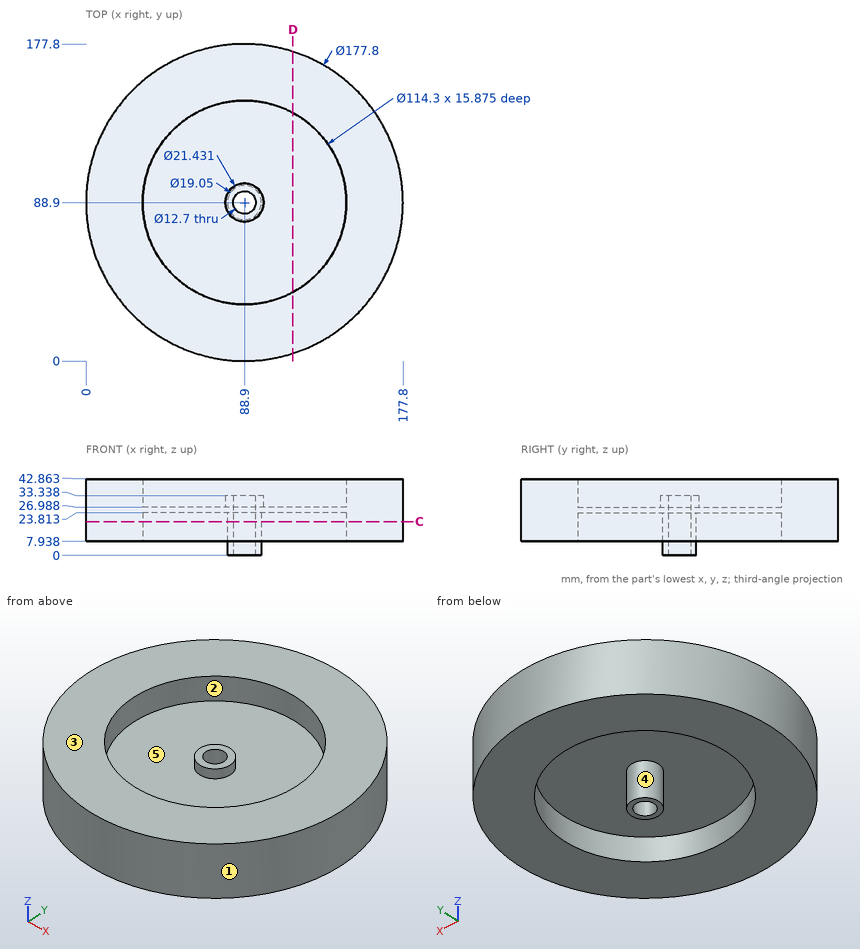
Geometry check sheet. Reference: drawing and pictorial views, mm from the part's lowest x, y, z. A direction names the side the tool comes from. Coordinates: 2 decimals unless noted, no trailing zeros. Loops run counter-clockwise (first coordinate to the right, second up) from the corner with the lowest first, then second, coordinate; pieces in that order, holes last. Notation, with made-up numbers: (-16, 60.5) -> (-7, 60.5) arc R19 cw to (-7, 68.5) -> close; hole circle Ø3 at (48, 83.5). An arc over 180 degrees is marked (long way). Write item = value, one per line. Start each with the question number.
1. Material ranges on line 1 (X direction, y = 88, z = 35) (1 decimal); line 2 (X direction, y = 88, z = 17) (1 decimal); line 3 (Y direction, x = 88.9, z = 33.5), recorded low to high.
2. Tool access check on the marked faces 4 and 5. Record the directions out of +Z, -Z, +X, -X, +Y, -Y that give a thin tool (end or side, any length) a straight path to the whole face; none if there is none.
3. Depth check by flat-ended pin: P1, Ø1, axis at y = 41, z = 11.5, coming from the -X side; P2, Ø8, axis at x = 76, z = 20.5, coming from the +Y side; P3, Ø5, axis at x = 48, y = 50, coming from the -Z side. Enter the tip coordinate at first touch or a pass-through.
4. Section check C-C on z = 19. Give the number of separate pieces and of enclosed holes in the cut face, then the cut area to 3 significant figures.
5. Section check D-D on x = 116. Record the cut outline in (y, z), then the cut area to 3 significant figures.
6. Draft check along X on the marked faces 1, 2 and 3. Enter one of: released by +X, released by -X, zero draft, split by the parting line, or undercut.
Responses:
q1.line_1 = 0 to 31.8, 146 to 177.8
q1.line_2 = 0 to 31.8, 79.4 to 82.6, 95.2 to 98.4, 146 to 177.8
q1.line_3 = 0 to 31.75, 146.05 to 177.8
q2.face_4 = -Z
q2.face_5 = +Z
q3.P1 = 13.69
q3.P2 = 177.35
q3.P3 = 7.94
q4.separate_pieces = 2
q4.enclosed_holes = 2
q4.area = 14,700 mm2
q5.outline = (4.23, 7.94) -> (38.58, 7.94) -> (38.58, 23.81) -> (139.22, 23.81) -> (139.22, 7.94) -> (173.57, 7.94) -> (173.57, 42.86) -> (139.22, 42.86) -> (139.22, 26.99) -> (38.58, 26.99) -> (38.58, 42.86) -> (4.23, 42.86) -> close
q5.area = 2,720 mm2
q6.face_1 = split by the parting line
q6.face_2 = undercut
q6.face_3 = zero draft
